Can you work these out from the model? Positions are in its coordinate system, mm. A direction names the side the tool comes from. Coordinates: 2 decimals unless noted, no trailing zeros. Order: outer loops, then holes, each group sorted by start corner. A loop starts at its lowest first (then second) coordinate and runs counter-clockwise, first axis right, second up. Notation, with made-up numbers: (-17.75, 13) -> (2.25, 13) arc R32 ccw to (2.25, 45) -> close; hole circle Ø4 at (72.25, 12.25). An arc over 180 degrees is marked (long way). Write item = value, one per line.
```python
from build123d import *

# Parameters (mm, degrees)
SKETCH1_R           = 22.5
BOSS_EXTRUDE1_DEPTH = 2
SKETCH2_R           = 8
BOSS_EXTRUDE2_DEPTH = 8
SKETCH3_R           = 2.5
CUT_EXTRUDE1_DEPTH  = 34.35416016
SKETCH4_R           = 3.6
CUT_EXTRUDE2_DEPTH  = 2.6
SKETCH5_R           = 1.25
CUT_EXTRUDE3_DEPTH  = 33.810059433
SKETCH7_W           = 7.216965313
SKETCH7_H           = 2
CUT_EXTRUDE4_DEPTH  = 10
CIRPATTERN1_COUNT   = 18


with BuildPart() as part:
    # Sketch1 → Boss-Extrude1 (new body)
    with BuildSketch(Plane.XY):
        Circle(SKETCH1_R)
    extrude(amount=BOSS_EXTRUDE1_DEPTH)

    # Sketch2 → Boss-Extrude2 (add)
    with BuildSketch(Plane.XY.offset(2)):
        Circle(SKETCH2_R)
    extrude(amount=BOSS_EXTRUDE2_DEPTH)

    # Sketch3 → Cut-Extrude1 (cut, through all)
    with BuildSketch(Plane.XY.offset(10)):
        Circle(SKETCH3_R)
    extrude(amount=-CUT_EXTRUDE1_DEPTH, mode=Mode.SUBTRACT)

    # Sketch4 → Cut-Extrude2 (cut)
    with BuildSketch(Plane.XY.offset(10)):
        Circle(SKETCH4_R)
    extrude(amount=-CUT_EXTRUDE2_DEPTH, mode=Mode.SUBTRACT)

    # Sketch5 → Cut-Extrude3 (cut, through all)
    with BuildSketch(Plane.XY.offset(2)):
        with Locations((0, 12)):
            Circle(SKETCH5_R)
        with Locations((-10.392304845, -6)):
            Circle(SKETCH5_R)
        with Locations((10.392304845, -6)):
            Circle(SKETCH5_R)
    extrude(amount=-CUT_EXTRUDE3_DEPTH, mode=Mode.SUBTRACT)

    # Sketch7 → Cut-Extrude4 (cut)
    with BuildSketch(Plane.XY.offset(2)):
        with Locations((19.628882318, 0)):
            Rectangle(SKETCH7_W, SKETCH7_H)
    cut_extrude4 = extrude(amount=-CUT_EXTRUDE4_DEPTH, mode=Mode.SUBTRACT)

    # CirPattern1: Cut-Extrude4 ×18 about axis
    cirpattern1_axis = Axis((0, 0, 0), (0, 0, 1))
    for i in range(1, CIRPATTERN1_COUNT):
        add(cut_extrude4.rotate(cirpattern1_axis, i * 360 / CIRPATTERN1_COUNT), mode=Mode.SUBTRACT)


solid = part.part
```
Item 1: I want a section at A-A, the plane y = 0. Please give me the cut outline in (x, z).
A:
outline = (-16.02, 0) -> (-2.5, 0) -> (-2.5, 7.4) -> (-3.6, 7.4) -> (-3.6, 10) -> (-8, 10) -> (-8, 2) -> (-16.02, 2) -> close; (2.5, 0) -> (16.02, 0) -> (16.02, 2) -> (8, 2) -> (8, 10) -> (3.6, 10) -> (3.6, 7.4) -> (2.5, 7.4) -> close
Item 2: I want a section at C-C, the plane y = 12. Please give me the cut outline in (x, z).
A:
outline = (-19.03, 0) -> (-15.86, 0) -> (-15.86, 2) -> (-19.03, 2) -> close; (-12.75, 0) -> (-1.25, 0) -> (-1.25, 2) -> (-12.75, 2) -> close; (1.25, 0) -> (12.75, 0) -> (12.75, 2) -> (1.25, 2) -> close; (15.86, 0) -> (19.03, 0) -> (19.03, 2) -> (15.86, 2) -> close
Item 3: If we mould it in two halves opening along X, with no side actions, what happens to faces 5 (the flat face through (-2.35, 19.09, 1.01)), 6 (the cylindrical face through (22.165, 3.867, 0.986)), 7 (the cylindrical face through (0, -22.5, 1)), 8 (the flat face through (8.02, 13.87, 1.01))? For each: pulls with the +X half, pulls with the -X half, needs draft (parallel to the pull), parting line crosses it, or undercut.
A:
face_5 = undercut
face_6 = pulls with the +X half
face_7 = parting line crosses it
face_8 = undercut
Item 4: For faces 1 (the flat face through (-19, 1, 1)), 2 (the flat face through (16.02, 0, 1)), 3 (the flat face through (18.39, -5.63, 1.01)), 4 (the flat face through (4.32, 18.74, 1.01)), which set-ups out of +Z, -Z, +X, -X, +Y, -Y let a thin tool reach every point of the face, with its end or its side?
A:
face_1 = +Z, -Z, -X
face_2 = +Z, -Z, +X
face_3 = +Z, -Z
face_4 = +Z, -Z, +Y
Item 5: I want a section at B-B, the plane x = 0. Please give me the cut outline in (y, z), plus the area to 3 significant figures.
A:
outline = (-22.5, 0) -> (-2.5, 0) -> (-2.5, 7.4) -> (-3.6, 7.4) -> (-3.6, 10) -> (-8, 10) -> (-8, 2) -> (-22.5, 2) -> close; (2.5, 0) -> (10.75, 0) -> (10.75, 2) -> (8, 2) -> (8, 10) -> (3.6, 10) -> (3.6, 7.4) -> (2.5, 7.4) -> close; (13.25, 0) -> (22.5, 0) -> (22.5, 2) -> (13.25, 2) -> close
area = 157 mm2
Item 6: If I drill on probe 1 along Y at (x, z) = (0, 0.6); probe 2 along Z at (x, y) = (8.5, -7); probe 3 along Y at (x, z) = (1.5, 5.5), over which ranges is the centre line in solid material (lowest first)?
A:
probe_1 = -22.5 to -2.5, 2.5 to 10.75, 13.25 to 22.5
probe_2 = 0 to 2
probe_3 = -7.86 to -2, 2 to 7.86
Item 7: I want a section at D-D, the plane z = 1. Give the number of separate pieces and of enclosed holes in the cut face, plus the area to 3 significant figures.
A:
separate_pieces = 1
enclosed_holes = 4
area = 1,320 mm2
Item 8: I'm going to push flat-ended pins straight in: P1, Ø1.6, axis at y = 0, z = 1, coming from the -X side; P2, Ø3, axis at x = 0, y = 12, coming from the -Z side; P3, Ø1.5, axis at x = -10.39, y = -6, coming from the -Z side; P4, Ø2, axis at x = 19.5, z = 1.5, coming from the +Y side. Where does each tip first touch, or does it pass through?
A:
P1 = -16.02
P2 = 0
P3 = through
P4 = 12.81
